Check sheet for the modelled part. Datum: model origin and axes. Units: mm. Face numbers are marked on the shaded views. A direction names the side the tool comes from. Round coordinates to 2 decimals unless told otherwise and drop trailing zeros. Write each loop counter-clockwise with the first axis right and the second up, starting at its lowest first coordinate (ties: lowest second). Pieces come first, ordered by that corner, then holes. Notation, with made-up numbers: (14, 80) -> (73, 80) arc R19 ccw to (73, 96) -> close; hole circle Ø1 at (-35.75, -6). An arc over 180 degrees is marked (long way). One line per item, written item: value.
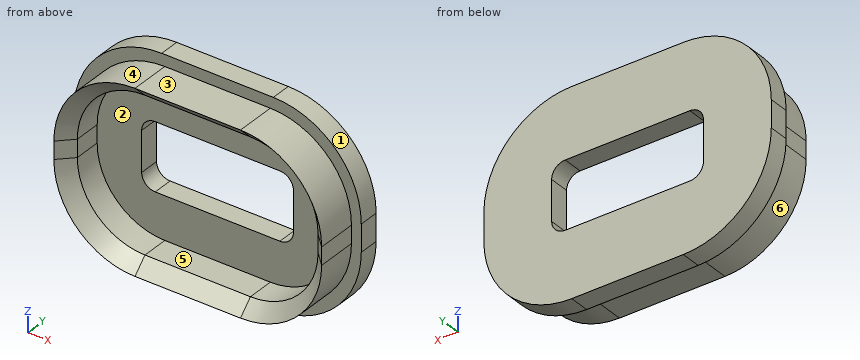
from build123d import *

# Parameters (mm, degrees)
F1_DEPTH = 3.81
F3_DEPTH = 7.62
F5_DEPTH = 3.811
F6_SIZE  = 2.53999


# Not quite as in the source:
# - a fillet or chamfer is up to 0.001 mm smaller than in the source, because OpenCascade refuses the exact size


with BuildPart() as f1:
    # F0 (on Front) → F1 (new body)
    with BuildSketch(Plane.XZ):
        with BuildLine():
            ThreePointArc((-26.9875, -2.54), (-22.1518329574, -14.2143329574), (-10.4775, -19.05))
            Line((-10.4775, -19.05), (10.4775, -19.05))
            ThreePointArc((10.4775, -19.05), (22.1518329574, -14.2143329574), (26.9875, -2.54))
            Line((26.9875, -2.54), (26.9875, 2.54))
            ThreePointArc((26.9875, 2.54), (22.1518329574, 14.2143329574), (10.4775, 19.05))
            Line((10.4775, 19.05), (-10.4775, 19.05))
            ThreePointArc((-10.4775, 19.05), (-22.1518329574, 14.2143329574), (-26.9875, 2.54))
            Line((-26.9875, 2.54), (-26.9875, -2.54))
        make_face()
    extrude(amount=F1_DEPTH)

    # F2 (on face) → F3 (join)
    with BuildSketch(Plane.XZ.offset(3.81)):
        with BuildLine():
            Line((9.906, 16.891), (-9.906, 16.891))
            ThreePointArc((-9.906, 16.891), (-20.6823073453, 12.4273073453), (-25.146, 1.651))
            Line((-25.146, 1.651), (-25.146, -1.651))
            ThreePointArc((-25.146, -1.651), (-20.6823073453, -12.4273073453), (-9.906, -16.891))
            Line((-9.906, -16.891), (9.906, -16.891))
            ThreePointArc((9.906, -16.891), (20.6823073453, -12.4273073453), (25.146, -1.651))
            Line((25.146, -1.651), (25.146, 1.651))
            ThreePointArc((25.146, 1.651), (20.6823073453, 12.4273073453), (9.906, 16.891))
        make_face()
        with BuildLine():
            Line((9.906, -14.351), (-9.906, -14.351))
            ThreePointArc((-9.906, -14.351), (-18.8862561211, -10.6312561211), (-22.606, -1.651))
            Line((-22.606, -1.651), (-22.606, 1.651))
            ThreePointArc((-22.606, 1.651), (-18.8862561211, 10.6312561211), (-9.906, 14.351))
            Line((-9.906, 14.351), (9.906, 14.351))
            ThreePointArc((9.906, 14.351), (18.8862561211, 10.6312561211), (22.606, 1.651))
            Line((22.606, 1.651), (22.606, -1.651))
            ThreePointArc((22.606, -1.651), (18.8862561211, -10.6312561211), (9.906, -14.351))
        make_face(mode=Mode.SUBTRACT)
    extrude(amount=F3_DEPTH)

    # F4 (on face) → F5 (cut, through all)
    with BuildSketch(Plane.XZ.offset(3.81)):
        with BuildLine():
            ThreePointArc((-14.2494, -3.7719), (-13.5054512242, -5.5679512242), (-11.7094, -6.3119))
            Line((-11.7094, -6.3119), (11.7094, -6.3119))
            ThreePointArc((11.7094, -6.3119), (13.5054512242, -5.5679512242), (14.2494, -3.7719))
            Line((14.2494, -3.7719), (14.2494, 3.7719))
            ThreePointArc((14.2494, 3.7719), (13.5054512242, 5.5679512242), (11.7094, 6.3119))
            Line((11.7094, 6.3119), (-11.7094, 6.3119))
            ThreePointArc((-11.7094, 6.3119), (-13.5054512242, 5.5679512242), (-14.2494, 3.7719))
            Line((-14.2494, 3.7719), (-14.2494, -3.7719))
        make_face()
    extrude(amount=-F5_DEPTH, mode=Mode.SUBTRACT)

    # F6 (size 2.54 in the source; OpenCascade refuses exactly that, so slightly less here)
    f6_edges = [f1.edges().sort_by_distance(p)[0] for p in [
        (-18.886256, -11.43, 10.631256),
        (0, -11.43, 14.351),
        (18.886256, -11.43, 10.631256),
        (18.886256, -11.43, -10.631256),
        (-18.886256, -11.43, -10.631256),
        (0, -11.43, -14.351),
        (22.606, -11.43, 0),
        (-22.606, -11.43, 0),
    ]]
    chamfer(f6_edges, length=F6_SIZE)


solid = f1.part
Item 1: Tool access check on the marked faces 4, 5 and 6. Record the directions out of +Z, -Z, +X, -X, +Y, -Y that give a thin tool (end or side, any length) a straight path to the whole face; none if there is none.
Answer:
face 4: +Z, -X, -Y
face 5: -Y
face 6: -Z, -X, -Y
Item 2: Depth check by flat-ended pin: P1, Ø19, axis at x = 11, z = -4.5, coming from the -Y side; P2, Ø1.5, axis at x = 5, y = -5.5, coming from the +Z side; P3, Ø3.5, axis at y = -6.5, z = -1, coming from the +X side; P4, Ø4, axis at x = 1.5, z = -2.5, coming from the +Y side. Enter the tip coordinate at first touch or a pass-through.
Answer:
P1: stops at y = -3.81
P2: stops at z = 16.89
P3: stops at x = 25.15
P4: passes through
Item 3: Mould release check, pull along X, two halves, no side actions. Record for the marked faces 1, 2 and 3: pulls with the +X half, pulls with the -X half, needs draft (parallel to the pull), parting line crosses it, or undercut.
Answer:
face 1: pulls with the +X half
face 2: undercut
face 3: needs draft
Item 4: Thickness scan on line 1 (X direction, y = -3.25, z = -3); line 2 (Z direction, x = -11, y = -1.5); line 3 (X direction, y = -6, z = 1). Record the ranges inside material, lowest first.
Answer:
line 1: x = -26.98 to -14.25, 14.25 to 26.98
line 2: z = -19.04 to -6.31, 6.31 to 19.04
line 3: x = -25.15 to -22.61, 22.61 to 25.15
Item 5: Sectioned sample at B-B on y = -2. Enter the section's corners in (x, z), and give its area (3 significant figures).
Answer:
outline: (-26.99, -2.54) arc R16.51 ccw to (-10.48, -19.05) -> (10.48, -19.05) arc R16.51 ccw to (26.99, -2.54) -> (26.99, 2.54) arc R16.51 ccw to (10.48, 19.05) -> (-10.48, 19.05) arc R16.51 ccw to (-26.99, 2.54) -> close; hole (-14.25, -3.77) arc R2.54 ccw to (-11.71, -6.31) -> (11.71, -6.31) arc R2.54 ccw to (14.25, -3.77) -> (14.25, 3.77) arc R2.54 ccw to (11.71, 6.31) -> (-11.71, 6.31) arc R2.54 ccw to (-14.25, 3.77) -> close
area: 1,470 mm^2
Item 6: Sectioned sample at C-C on y = -7.5. Enter the section's corners in (x, z), and give its area (3 significant figures).
Answer:
outline: (-25.15, -1.65) arc R15.24 ccw to (-9.91, -16.89) -> (9.91, -16.89) arc R15.24 ccw to (25.15, -1.65) -> (25.15, 1.65) arc R15.24 ccw to (9.91, 16.89) -> (-9.91, 16.89) arc R15.24 ccw to (-25.15, 1.65) -> close; hole (-22.61, -1.65) arc R12.7 ccw to (-9.91, -14.35) -> (9.91, -14.35) arc R12.7 ccw to (22.61, -1.65) -> (22.61, 1.65) arc R12.7 ccw to (9.91, 14.35) -> (-9.91, 14.35) arc R12.7 ccw to (-22.61, 1.65) -> close
area: 340 mm^2
